```python
from build123d import *

# Parameters (mm, degrees)
SKETCH1_W           = 20
SKETCH1_H           = 40
SKETCH1_R           = 1.1
SKETCH1_R_2         = 6.5
BOSS_EXTRUDE2_DEPTH = 4


with BuildPart() as part:
    # Sketch1 → Boss-Extrude2 (new body)
    with BuildSketch(Plane.XY):
        Rectangle(SKETCH1_W, SKETCH1_H)
        with Locations((7, -10)):
            Circle(SKETCH1_R, mode=Mode.SUBTRACT)
        with Locations((-6, -10.118141531)):
            Circle(SKETCH1_R, mode=Mode.SUBTRACT)
        with Locations((-8, 2.93366218)):
            Circle(SKETCH1_R, mode=Mode.SUBTRACT)
        with Locations((8, 3)):
            Circle(SKETCH1_R, mode=Mode.SUBTRACT)
        with Locations((0, 10)):
            Circle(SKETCH1_R_2, mode=Mode.SUBTRACT)
        with BuildLine():
            Line((-4, 23), (-4, 20))
            Line((-4, 20), (4, 20))
            Line((4, 20), (4, 23))
            ThreePointArc((4, 23), (3.707106781, 23.707106781), (3, 24))
            Line((3, 24), (-3, 24))
            ThreePointArc((-3, 24), (-3.707106781, 23.707106781), (-4, 23))
        make_face()
        with BuildLine():
            Line((11, 5.93366218), (10, 5.93366218))
            Line((10, 5.93366218), (10, -0.06633782))
            Line((10, -0.06633782), (11, -0.06633782))
            ThreePointArc((11, -0.06633782), (11.707106781, 0.226555399), (12, 0.93366218))
            Line((12, 0.93366218), (12, 4.93366218))
            ThreePointArc((12, 4.93366218), (11.707106781, 5.640768961), (11, 5.93366218))
        make_face()
        with BuildLine():
            Line((4, -20), (-4, -20))
            Line((-4, -20), (-4, -23))
            ThreePointArc((-4, -23), (-3.707106781, -23.707106781), (-3, -24))
            Line((-3, -24), (3, -24))
            ThreePointArc((3, -24), (3.707106781, -23.707106781), (4, -23))
            Line((4, -23), (4, -20))
        make_face()
        with BuildLine():
            Line((-10, -0.06633782), (-10, 5.93366218))
            Line((-10, 5.93366218), (-11, 5.93366218))
            ThreePointArc((-11, 5.93366218), (-11.707106781, 5.640768961), (-12, 4.93366218))
            Line((-12, 4.93366218), (-12, 0.93366218))
            ThreePointArc((-12, 0.93366218), (-11.707106781, 0.226555399), (-11, -0.06633782))
            Line((-11, -0.06633782), (-10, -0.06633782))
        make_face()
    extrude(amount=BOSS_EXTRUDE2_DEPTH)


solid = part.part
```
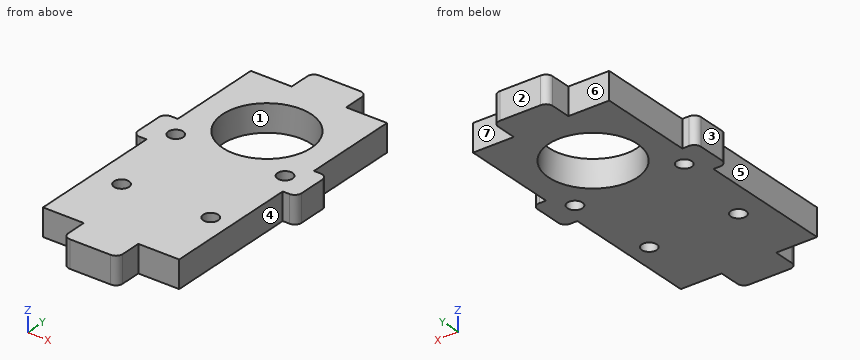
Model file for the job. Use its own axes, mm. Face numbers are marked on the shaded views. A direction names the side the tool comes from. Give positions to 0.01 mm unless a question says otherwise; leave off trailing zeros. Loops run counter-clockwise (first coordinate to the right, second up) from the corner with the lowest first, then second, coordinate; pieces in that order, holes last. Notation, with made-up numbers: (-37.75, 9.5) - (-10.75, 9.5) arc R10 cw to (-10.75, 21.5) - close; hole circle Ø9 at (24, -7.5). An arc over 180 degrees is marked (long way). One line per item, written item: value. Start each with the question number.
1. Probe L1, parallel to X at y = -9.5, z = 3.7; L2, parallel to Y at x = 7, z = 1.1; L3, parallel to Y at x = 7.75, z = 1.5. List the from-to ranges inside material, lowest first. Write a range as from..to.
2. Which spindle directions (+Z, -Z, +X, -X, +Y, -Y) get a long thin tool onto all of the face, cutting with end or side? Do the marked faces 4, 5, 6 and 7. Say none if no direction does.
3. Slice it at C-C (z = 2.35). Give the number of separate pieces and of enclosed holes in the cut face, plus the area to 3 significant figures.
4. Slice it at A-A (x = -6). List the corners of the cut face in (y, z).
5. Slice it at D-D (y = -21). List the corners of the cut face in (x, z), plus the area to 3 significant figures.
6. Pull direction Y, two halves, no side cores. Call the marked faces 1, 2 and 3: pulls with the +Y half, pulls with the -Y half, needs draft (parallel to the pull), parting line crosses it, or undercut.
7. Pin check, flat tips, straight feed: pin 1 (2 mm diameter, centred on x = -8, z = 2.5, fed in from +Y); pin 2 (0.5 mm diameter, centred on x = -10.5, z = 1.5, fed in from -Y); pin 3 (1.3 mm diameter, centred on x = 8, y = 3, fed in from -Z); pin 4 (1.5 mm diameter, centred on y = 21.5, z = 2, fed in from +X). Stop position of each tip, or through.
8. Slice it at B-B (x = 1.25). List the corners of the cut face in (y, z).
Solution:
1. L1: x = -10..-6.91, -5.09..6.02, 7.98..10
1. L2: y = -20..-11.1, -8.9..2.54, 3.46..20
1. L3: y = -20..-10.8, -9.2..1.93, 4.07..20
2. face 4: +Z, -Z, +X, -Y
2. face 5: +Z, -Z, -X, -Y
2. face 6: +Z, -Z, -X, +Y
2. face 7: +Z, -Z, +X, +Y
3. separate pieces: 1
3. enclosed holes: 5
3. area: 738 mm^2
4. outline: (-20, 0) - (-11.22, 0) - (-11.22, 4) - (-20, 4) - close; (-9.02, 0) - (7.5, 0) - (7.5, 4) - (-9.02, 4) - close; (12.5, 0) - (20, 0) - (20, 4) - (12.5, 4) - close
5. outline: (-4, 0) - (4, 0) - (4, 4) - (-4, 4) - close
5. area: 32.0 mm^2
6. face 1: undercut
6. face 2: pulls with the +Y half
6. face 3: needs draft
7. pin 1: stops at y = 20
7. pin 2: stops at y = -0.07
7. pin 3: passes through
7. pin 4: stops at x = 4
8. outline: (-24, 0) - (3.62, 0) - (3.62, 4) - (-24, 4) - close; (16.38, 0) - (24, 0) - (24, 4) - (16.38, 4) - close
